Geometry check sheet. Reference: the model listing, model coordinates, mm. A direction names the side the tool comes from. Round coordinates to 2 decimals unless told otherwise and drop trailing zeros. Write each loop counter-clockwise with the first axis right and the second up, starting at its lowest first coordinate (ties: lowest second). Pieces come first, ordered by that corner, then holes. Notation, with made-up numbers: M -21,42.25 L 11,42.25 A17 cw 11,73.25 Z; hole C 2.25,0.5 d8. An arc over 180 degrees is marked long. Answer as CSV lines item,"result". Start each with the question number.
```python
from build123d import *

# Parameters (mm, degrees)
UPN_UPN180_1_DEPTH = 210
SKETCH17_R         = 15
CUT_EXTRUDE1_DEPTH = 10
FILLET1_R          = 2


with BuildPart() as part:
    # Sketch110 → Upn UPN180(1) (new body)
    with BuildSketch(Plane(origin=(0, 186.578947368, 0), x_dir=(0, 0, -1), z_dir=(0, -1, 0))):
        with BuildLine():
            Line((70, 180), (0, 180))
            Line((0, 180), (0, 0))
            Line((0, 0), (70, 0))
            Line((70, 0), (70, 3.122386663))
            ThreePointArc((70, 3.122386663), (68.541183887, 6.853181859), (64.938606257, 8.604870092))
            Line((64.938606257, 8.604870092), (18.122787486, 12.350200343))
            ThreePointArc((18.122787486, 12.350200343), (10.917632226, 15.85357681), (8, 23.315167202))
            Line((8, 23.315167202), (8, 156.684832798))
            ThreePointArc((8, 156.684832798), (10.917632226, 164.14642319), (18.122787486, 167.649799657))
            Line((18.122787486, 167.649799657), (64.938606257, 171.395129908))
            ThreePointArc((64.938606257, 171.395129908), (68.541183887, 173.146818141), (70, 176.877613337))
            Line((70, 176.877613337), (70, 180))
        make_face()
    extrude(amount=UPN_UPN180_1_DEPTH)

    # Sketch17 → Cut-Extrude1 (cut)
    with BuildSketch(Plane(origin=(0, 0, -8), x_dir=(-1, 0, 0), z_dir=(0, 0, -1))):
        with Locations((-90, 126.578947368)):
            Circle(SKETCH17_R)
    extrude(amount=-CUT_EXTRUDE1_DEPTH, mode=Mode.SUBTRACT)

    # Fillet1
    fillet1_edges = [part.edges().sort_by_distance(p)[0] for p in [
        (169.522464782, 186.578947368, -41.530696872),
        (164.14642319, 186.578947368, -10.917632226),
        (180, -23.421052632, -35),
        (90, 186.578947368, -8),
        (15.85357681, 186.578947368, -10.917632226),
        (10.477535218, 186.578947368, -41.530696872),
        (6.853181859, 186.578947368, -68.541183887),
        (1.561193332, 186.578947368, -70),
        (0, 186.578947368, -35),
        (90, 186.578947368, 0),
        (180, 186.578947368, -35),
        (178.438806668, 186.578947368, -70),
        (173.146818141, 186.578947368, -68.541183887),
        (90, -23.421052632, 0),
        (0, -23.421052632, -35),
        (0, 81.578947368, -70),
        (0, 81.578947368, 0),
        (180, 81.578947368, 0),
        (180, 81.578947368, -70),
        (1.561193332, -23.421052632, -70),
        (6.853181859, -23.421052632, -68.541183887),
        (10.477535218, -23.421052632, -41.530696872),
        (15.85357681, -23.421052632, -10.917632226),
        (90, -23.421052632, -8),
        (164.14642319, -23.421052632, -10.917632226),
        (169.522464782, -23.421052632, -41.530696872),
        (173.146818141, -23.421052632, -68.541183887),
        (178.438806668, -23.421052632, -70),
    ]]
    fillet(fillet1_edges, radius=FILLET1_R)


solid = part.part
```
1) Scan lines: line 1 (Y direction, x = 90, z = -3); line 2 (Z direction, x = 121, y = 88.5); line 3 (X direction, y = 122, z = -10). Record each from-to range of solid material in increasing order. Write a range as from..to.
2) Section check B-B, the plane y = 133. Record the cut outline in (x, z), plus the area to 3 significant figures.
3) Mould release check, pull along X, two halves, no side actions. Record for faces 1 (the flat face through (0, 83, -35)), 2 (the cylindrical face through (170.15, -22.85, -41.81)), 3 (the flat face through (91, 83, 0)): released by +X, released by -X, zero draft, split by the parting line, or undercut.
4) Section check C-C, the plane x = 28.5. Record the cut outline in (y, z), plus the area to 3 significant figures.
5) Section check D-D, the plane y = 97.5. Record the cut outline in (x, z), plus the area to 3 significant figures.
6) Section check A-A, the plane x = 90. Record the cut outline in (y, z).
7) Access from +Z, -Z, +X, -X, +Y, -Y to the whole of each face (thin tool, end or side, straight path). Record for faces 4 (the flat face through (10.45, 83.02, -41.86)), 5 (the cylindrical face through (9.904, -22.851, -41.155)), 6 (the cylindrical face through (9.9, 186.01, -41.16)).
Results:
1,line 1,"y = -23.42..111.58, 141.58..186.58"
1,line 2,"z = -8..0"
1,line 3,"x = 0..16.99, 163.01..180"
2,outline,"M 0,-68 A2 ccw 2,-70 L 3.12,-70 A5.5 ccw 8.6,-64.94 L 12.35,-18.12 A11 cw 23.32,-8 L 76.44,-8 L 76.44,0 L 2,0 A2 ccw 0,-2 Z; M 103.56,-8 L 156.68,-8 A11 cw 167.65,-18.12 L 171.4,-64.94 A5.5 ccw 176.88,-70 L 178,-70 A2 ccw 180,-68 L 180,-2 A2 ccw 178,0 L 103.56,0 Z"
2,area,"2,580 mm^2"
3,face 1,"released by -X"
3,face 2,"undercut"
3,face 3,"zero draft"
4,outline,"M -23.42,-6 A2 ccw -21.42,-8 L 184.58,-8 A2 ccw 186.58,-6 L 186.58,-2 A2 ccw 184.58,0 L -21.42,0 A2 ccw -23.42,-2 Z"
4,area,"1,680 mm^2"
5,outline,"M 0,-68 A2 ccw 2,-70 L 3.12,-70 A5.5 ccw 8.6,-64.94 L 12.35,-18.12 A11 cw 23.32,-8 L 156.68,-8 A11 cw 167.65,-18.12 L 171.4,-64.94 A5.5 ccw 176.88,-70 L 178,-70 A2 ccw 180,-68 L 180,-2 A2 ccw 178,0 L 2,0 A2 ccw 0,-2 Z"
5,area,"2,790 mm^2"
6,outline,"M -23.42,-6 A2 ccw -21.42,-8 L 111.58,-8 L 111.58,0 L -21.42,0 A2 ccw -23.42,-2 Z; M 141.58,-8 L 184.58,-8 A2 ccw 186.58,-6 L 186.58,-2 A2 ccw 184.58,0 L 141.58,0 Z"
7,face 4,"-Z, +Y, -Y"
7,face 5,"-Z, -Y"
7,face 6,"-Z, +Y"
